Geometry check sheet. Reference: the model listing, model coordinates, mm. A direction names the side the tool comes from. Coordinates: 2 decimals unless noted, no trailing zeros. Write each loop counter-clockwise with the first axis right and the second up, starting at its lowest first coordinate (ties: lowest second). Pieces come first, ordered by that corner, then holes.
from build123d import *

# Parameters (mm, degrees)
SKETCH009_W             = 84
SKETCH009_H             = 70
PAD002_DEPTH            = 2
SKETCH010_W             = 2
SKETCH010_H             = 7
PAD003_DEPTH            = 2
SKETCH012_W             = 8
SKETCH012_H             = 6.8
PAD004_DEPTH            = 4
SKETCH013_W             = 7
SKETCH013_H             = 6
PAD005_DEPTH            = 4
SKETCH011_W             = 8
SKETCH011_H             = 6.8
PAD006_DEPTH            = 4
SKETCH014_R             = 1.15
POCKET002_DEPTH         = 81.001
SKETCH016_R             = 1.15
POCKET003_DEPTH         = 8.501
SKETCH018_W             = 11.5
SKETCH018_H             = 11.5
POCKET004_DEPTH         = 5
POCKET005_DEPTH         = 5
POCKET006_DEPTH         = 5
SKETCH021_W             = 1
SKETCH021_H             = 7
PAD007_DEPTH            = 1
SKETCH022_W             = 9
SKETCH022_H             = 10
POCKET007_DEPTH         = 0.4
FILLET_R                = 3
BODY002_PITCH_ANGLE     = -90
BODY002_PLACEMENT_ANGLE = 90
PAD001_DEPTH            = 35
SKETCH007_W             = 11.5
SKETCH007_H             = 11.5
POCKET001_DEPTH         = 13
FILLET001_R             = 3
SKETCH025_W             = 6.5
SKETCH025_H             = 9
SKETCH025_W_2           = 9
SKETCH025_H_2           = 6.5
POCKET008_DEPTH         = 8


with BuildPart() as back:
    # Sketch009 → Pad002 (new body)
    with BuildSketch(Plane.XY):
        Rectangle(SKETCH009_W, SKETCH009_H)
    extrude(amount=PAD002_DEPTH)

    # Sketch010 (on Face6 of Pad002) → Pad003 (join)
    with BuildSketch(Plane.XY.offset(2)):
        with Locations((-38, -1)):
            Rectangle(SKETCH010_W, SKETCH010_H)
        Polygon((-21, 32), (39, 32), (39, -4), (37, -4), (37, 30), (-21, 30), align=None)
    extrude(amount=PAD003_DEPTH)

    # Sketch012 (on Face15 of Pad003) → Pad004 (join)
    with BuildSketch(Plane.YZ.offset(39)):
        with Locations((0, 5.4)):
            Rectangle(SKETCH012_W, SKETCH012_H)
    extrude(amount=-PAD004_DEPTH)

    # Sketch013 (on Face9 of Pad004) → Pad005 (join)
    with BuildSketch(Plane(origin=(-39, 0, 0), x_dir=(0, -1, 0), z_dir=(-1, 0, 0))):
        with Locations((1, 5)):
            Rectangle(SKETCH013_W, SKETCH013_H)
    extrude(amount=-PAD005_DEPTH)

    # Sketch011 (on Face16 of Pad003) → Pad006 (join)
    with BuildSketch(Plane(origin=(0, 32, 0), x_dir=(-1, 0, 0), z_dir=(0, 1, 0))):
        with Locations((-29, 5.4)):
            Rectangle(SKETCH011_W, SKETCH011_H)
        with Locations((14, 5.4)):
            Rectangle(SKETCH011_W, SKETCH011_H)
    extrude(amount=-PAD006_DEPTH)

    # Sketch014 (on Face44 of Pad006) → Pocket002 (cut, through all)
    with BuildSketch(Plane.YZ.offset(39)):
        with Locations((0, 5)):
            Circle(SKETCH014_R)
    extrude(amount=-POCKET002_DEPTH, mode=Mode.SUBTRACT)

    # Sketch016 → Pocket003 (cut, through all)
    with BuildSketch(Plane.XZ.offset(-26.5)):
        with Locations((-13, 5)):
            Circle(SKETCH016_R)
        with Locations((30, 5)):
            Circle(SKETCH016_R)
    extrude(amount=-POCKET003_DEPTH, mode=Mode.SUBTRACT)

    # Sketch018 (on Face5 of Pocket003) → Pocket004 (cut)
    with BuildSketch(Plane.XY.offset(2)):
        with Locations((0, 17.75)):
            Rectangle(SKETCH018_W, SKETCH018_H)
    extrude(amount=-POCKET004_DEPTH, mode=Mode.SUBTRACT)

    # Sketch019 (on Face31 of Pocket004) → Pocket005 (cut)
    with BuildSketch(Plane.XZ.offset(-28)):
        Polygon((29.125944, 9.042901), (33.258869, 4.499726), (33.258869, 9.042901), align=None)
    extrude(amount=-POCKET005_DEPTH, mode=Mode.SUBTRACT)

    # Sketch020 (on Face36 of Pocket005) → Pocket006 (cut)
    with BuildSketch(Plane(origin=(35, 0, 0), x_dir=(0, -1, 0), z_dir=(-1, 0, 0))):
        Polygon((2.77547, 8.938441), (6.386171, 3.079567), (6.386171, 8.938441), align=None)
    extrude(amount=-POCKET006_DEPTH, mode=Mode.SUBTRACT)

    # Sketch021 (on Face40 of Pocket006) → Pad007 (join)
    with BuildSketch(Plane.XY.offset(8)):
        with Locations((-38.5, -1)):
            Rectangle(SKETCH021_W, SKETCH021_H)
    extrude(amount=PAD007_DEPTH)

    # Sketch022 (on Face5 of Pocket005) → Pocket007 (cut)
    with BuildSketch(Plane.XY.offset(2)):
        with Locations((-30.3, 30)):
            Rectangle(SKETCH022_W, SKETCH022_H)
    extrude(amount=-POCKET007_DEPTH, mode=Mode.SUBTRACT)

    # Fillet
    fillet_edges = [back.edges().sort_by_distance(p)[0] for p in [
        (42, 35, 1),
        (-42, 35, 1),
    ]]
    fillet(fillet_edges, radius=FILLET_R)


with BuildPart() as back_1:
    # Body002 pitch: moved
    add(back.part.rotate(Axis((0, 0, 0), (0, 1, 0)), BODY002_PITCH_ANGLE))


with BuildPart() as back_2:
    # Body002 placement: moved
    add(back_1.part.rotate(Axis((0, 0, 0), (0, 0, 1)), BODY002_PLACEMENT_ANGLE))


with BuildPart() as curve:
    # Sketch006 → Pad001 (new body, symmetric)
    with BuildSketch(Plane(origin=(0, 0, 0), x_dir=(0, 0, -1), z_dir=(1, 0, 0))):
        with BuildLine():
            ThreePointArc((-42, 3.4), (0, 0.756736), (42, 3.4))
            Line((42, -0.1), (42, 3.4))
            Line((-42, -0.1), (42, -0.1))
            Line((-42, 3.4), (-42, -0.1))
        make_face()
    extrude(amount=PAD001_DEPTH, both=True)

    # Sketch007 (on Face3 of Pad001) → Pocket001 (cut)
    with BuildSketch(Plane.XZ.offset(0.1)):
        with Locations((-17.75, 0)):
            Rectangle(SKETCH007_W, SKETCH007_H)
    extrude(amount=-POCKET001_DEPTH, mode=Mode.SUBTRACT)

    # Fillet001
    fillet001_edges = [curve.edges().sort_by_distance(p)[0] for p in [
        (-35, 1.65, -42),
        (-35, 1.65, 42),
    ]]
    fillet(fillet001_edges, radius=FILLET001_R)

    # Boolean: union Back
    add(back_2.part)

    # Sketch025 (on Face32 of Boolean) → Pocket008 (cut, symmetric)
    with BuildSketch(Plane.XZ.offset(2)):
        with Locations((-28.75, 0)):
            Rectangle(SKETCH025_W, SKETCH025_H)
        with Locations((-15.55, 13.625)):
            Rectangle(SKETCH025_W_2, SKETCH025_H_2)
        with Locations((-2.05, 0)):
            Rectangle(SKETCH025_W, SKETCH025_H)
        with Locations((-15.55, -13.625)):
            Rectangle(SKETCH025_W_2, SKETCH025_H_2)
    extrude(amount=POCKET008_DEPTH, both=True, mode=Mode.SUBTRACT)


solid = curve.part
1. Thickness scan on line 1 along Z through (x, y) = (3, -4.5); line 2 along Z through (x, y) = (-30.5, -4.25); line 3 along X through (y, z) = (-5, -36.55). Record the ranges inside material, lowest first.
Computed values:
line 1: z = -39 to -35, 35 to 39
line 2: z = -18 to -13.87, -12.13 to -10, 25 to 29.13, 30.87 to 33
line 3: x = -2.5 to -1.15, 1.15 to 4.5
2. Sectioned sample at D-D, the plane z = -13. Record the boundary of the cut face in (x, y).
Computed values:
outline: (-35, -2) - (-32, -2) - (-32, -3.85) - (-28, -3.85) - (-28, -2) - (-20.05, -2) - (-20.05, 1.01) - (-35, 1.01) - close; (-32, -8.8) - (-28, -8.8) - (-28, -6.15) - (-32, -6.15) - close; (-11.05, -2) - (35, -2) - (35, 1.01) - (-11.05, 1.01) - close
3. Access from +Z, -Z, +X, -X, +Y, -Y to the whole of each face (thin tool, end or side, straight path). Record for faces 1 (the flat face through (-31, -4, 15)), 2 (the flat face through (2, -5, -39)), 3 (the flat face through (-5.3, -1, 0)).
Computed values:
face 1: +X, -X, -Y
face 2: -Z, +X, -X, -Y
face 3: +Y, -Y
4. Gauge pin test, flat ends, axial feed: pin 1 Ø6 at (x, z) = (8, 10) entering from +Y; pin 2 Ø1 at (x, z) = (-31.5, -19) entering from -Y; pin 3 Ø1.2 at (x, y) = (-29.5, -6) entering from -Z; pin 4 Ø5 at (y, z) = (-7.5, -3) entering from +X. Record the tip position at first contact, or that the pin passes through.
Computed values:
pin 1: stops at y = 1.01
pin 2: stops at y = -4
pin 3: stops at z = -18
pin 4: passes through
5. Sectioned sample at A-A, the plane x = 0. Record the boundary of the cut face in (y, z).
Computed values:
outline: (-9, -39) - (-6.15, -39) - (-6.15, -35) - (-8, -35) - (-8, -38) - (-9, -38) - close; (-8.8, 35) - (-6.15, 35) - (-6.15, 39) - (-8.8, 39) - close; (-3.85, -39) - (-2, -39) - (-2, -42) - (3.4, -42) arc R335 cw to (0.79, -4.5) - (-2, -4.5) - (-2, -35) - (-3.85, -35) - close; (-3.85, 35) - (-2, 35) - (-2, 4.5) - (0.79, 4.5) arc R335 cw to (3.4, 42) - (-2, 42) - (-2, 39) - (-3.85, 39) - close
6. Sectioned sample at B-B, the plane x = -26.5. Record the boundary of the cut face in (y, z), and give its area (3 significant figures).
Computed values:
outline: (-4, 37) - (-2, 37) - (-2, 4.5) - (0.79, 4.5) arc R335 cw to (3.4, 42) - (-2, 42) - (-2, 39) - (-4, 39) - close; (-2, -42) - (3.4, -42) arc R335 cw to (0.79, -4.5) - (-2, -4.5) - (-2, -25.8) - (-1.6, -25.8) - (-1.6, -34.8) - (-2, -34.8) - close
area: 281 mm2
7. Sectioned sample at C-C, the plane y = -0.25. Record the boundary of the cut face in (x, z) (3 decimals).
Computed values:
outline: (-35, -39) arc R3 ccw to (-32, -42) - (35, -42) - (35, 42) - (-32, 42) arc R3 ccw to (-35, 39) - close; hole (-32, -4.5) - (-25.5, -4.5) - (-25.5, 4.5) - (-32, 4.5) - close; hole (-23.5, -5.75) - (-12, -5.75) - (-12, 5.75) - (-23.5, 5.75) - close; hole (-20.05, -16.875) - (-11.05, -16.875) - (-11.05, -10.375) - (-20.05, -10.375) - close; hole (-20.05, 10.375) - (-11.05, 10.375) - (-11.05, 16.875) - (-20.05, 16.875) - close; hole (-5.3, -4.5) - (1.2, -4.5) - (1.2, 4.5) - (-5.3, 4.5) - close
8. Draft check along Z on faces 4 (the flat face through (-31, -3, -21)), 5 (the flat face through (-31, -4, -19)), 6 (the flat face through (1.2, -1, 0)). Enter one of: released by +Z, released by -Z, zero draft, split by the parting line, or undercut.
Computed values:
face 4: released by -Z
face 5: zero draft
face 6: undercut
